```python
from build123d import *

# Parameters (mm, degrees)
F0_W           = 430
F0_H           = 340
F1_DEPTH       = 25
F2_T           = -2.5
F4_D           = 6
F4_DEPTH       = 1000
F4_CBORE_D     = 6
F4_CBORE_DEPTH = 5


with BuildPart() as f1:
    # F0 (on Top) → F1 (new body)
    with BuildSketch(Plane.XY):
        Rectangle(F0_W, F0_H)
    extrude(amount=F1_DEPTH)

    # F2
    f2_openings = [f1.faces().sort_by_distance(p)[0] for p in [
        (0, 0, 0),
        (0, -170, 12.5),
    ]]
    offset(amount=F2_T, openings=f2_openings)

    # F4
    with Locations(Plane(origin=(-215, 0, 0), x_dir=(0, -1, 0), z_dir=(-1, 0, 0))):
        with Locations((-85, 12.5), (85, 12.5)):
            CounterBoreHole(F4_D / 2, F4_CBORE_D / 2, F4_CBORE_DEPTH, depth=F4_DEPTH)


solid = f1.part
```
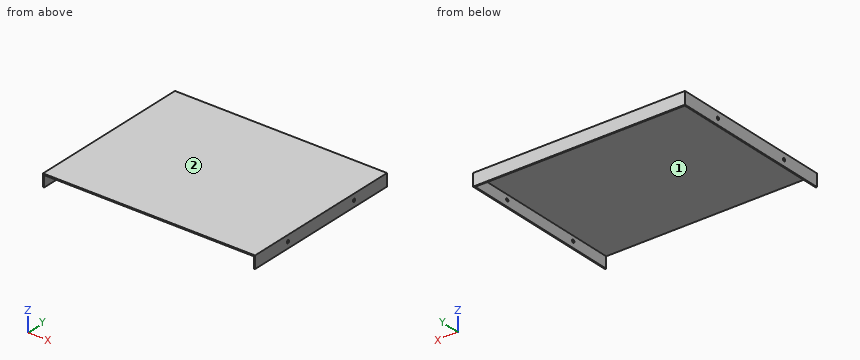
Here's how the part is built. I have some questions about the finished solid (model axes, mm). Face numbers are marked on the shaded views. Coordinates: 2 decimals unless noted, no trailing zeros. Order: outer loops, then holes, each group sorted by start corner. A loop starts at its lowest first (then second) coordinate and runs counter-clockwise, first axis right, second up.
1) Will these pins go through, and if not, where does the flat tip stop? pin 1 (8 mm diameter, centred on y = 85, z = 12.5, fed in from -X); pin 2 (6 mm diameter, centred on x = 148.5, y = 81, fed in from -Z); pin 3 (6 mm diameter, centred on x = -58, z = 12, fed in from -Y).
2) I need wall thicknesses on line 1 (Y direction, x = 214.35, z = 12.5); line 2 (Z direction, x = 213, y = -85); line 3 (X direction, y = 90, z = 20). Which ranges of each line are inside material? Lowest first, please.
3) Imagine slicing it at A-A on y = -109.5. List the corners of the cut face in (x, z) for me.
4) Imagine slicing it at B-B on x = -106. List the corners of the cut face in (y, z) for me.
5) We'd pull the mould along X, two halves only. Please class the marked faces 1 and 2: +X half, -X half, draft (parallel to the pull), parting line (faces both ways), or undercut.
Response values:
1. pin 1: stops at x = -215
1. pin 2: stops at z = 22.5
1. pin 3: stops at y = 167.5
2. line 1: y = -170 to -88, -82 to 82, 88 to 170
2. line 2: z = 0 to 9.5, 15.5 to 25
2. line 3: x = -215 to -212.5, 212.5 to 215
3. outline: (-215, 0) - (-212.5, 0) - (-212.5, 22.5) - (212.5, 22.5) - (212.5, 0) - (215, 0) - (215, 25) - (-215, 25) - close
4. outline: (-170, 22.5) - (167.5, 22.5) - (167.5, 0) - (170, 0) - (170, 25) - (-170, 25) - close
5. face 1: undercut
5. face 2: draft
